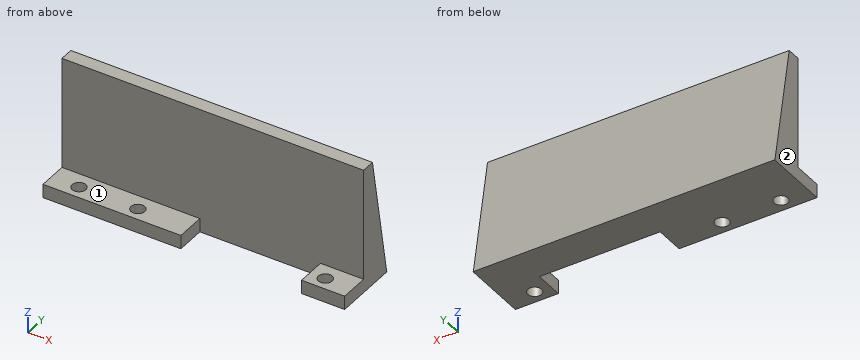
from build123d import *

# Parameters (mm, degrees)
SKETCH1_W           = 70
SKETCH1_H           = 26
BOSS_EXTRUDE1_DEPTH = 3.175
SKETCH2_W           = 70
SKETCH2_H           = 10
BOSS_EXTRUDE2_DEPTH = 3.175
SKETCH3_R           = 1.6
CUT_EXTRUDE1_DEPTH  = 3.175
BOSS_EXTRUDE3_DEPTH = 70
SKETCH5_W           = 28
SKETCH5_H           = 6.825
CUT_EXTRUDE2_DEPTH  = 10


with BuildPart() as part:
    # Sketch1 → Boss-Extrude1 (new body)
    with BuildSketch(Plane(origin=(0, 0, 0), x_dir=(1, 0, 0), z_dir=(0, 1, 0))):
        Rectangle(SKETCH1_W, SKETCH1_H)
    extrude(amount=BOSS_EXTRUDE1_DEPTH)

    # Sketch2 → Boss-Extrude2 (add)
    with BuildSketch(Plane(origin=(0, 0, -13), x_dir=(-1, 0, 0), z_dir=(0, 0, -1))):
        with Locations((0, -1.825)):
            Rectangle(SKETCH2_W, SKETCH2_H)
    extrude(amount=BOSS_EXTRUDE2_DEPTH)

    # Sketch3 → Cut-Extrude1 (cut)
    with BuildSketch(Plane.XY.offset(-13)):
        with Locations((-14.914, -3.825)):
            Circle(SKETCH3_R)
        with Locations((28.575, -3.825)):
            Circle(SKETCH3_R)
        with Locations((-28.575, -3.825)):
            Circle(SKETCH3_R)
    extrude(amount=-CUT_EXTRUDE1_DEPTH, mode=Mode.SUBTRACT)

    # Sketch4 → Boss-Extrude3 (add)
    with BuildSketch(Plane(origin=(35, 0, 0), x_dir=(0, 0, -1), z_dir=(1, 0, 0))):
        Polygon((16.175, 3.175), (16.175, 8.412812241), (16.143192443, 8.313731132), (-13, 3.175), align=None)
    extrude(amount=-BOSS_EXTRUDE3_DEPTH)

    # Sketch5 → Cut-Extrude2 (cut)
    with BuildSketch(Plane(origin=(0, 0, -16.175), x_dir=(-1, 0, 0), z_dir=(0, 0, -1))):
        with Locations((-11, -3.4125)):
            Rectangle(SKETCH5_W, SKETCH5_H)
    extrude(amount=-CUT_EXTRUDE2_DEPTH, mode=Mode.SUBTRACT)


solid = part.part
Could you check a few things on this model? Use its own coordinates, in mm. Face numbers are marked on the shaded views. A direction names the side the tool comes from. Round coordinates to 2 decimals unless told otherwise and drop trailing zeros. Write each loop counter-clockwise with the first axis right and the second up, starting at its lowest first coordinate (ties: lowest second). Pieces come first, ordered by that corner, then holes. Notation, with made-up numbers: (79.5, 49) -> (85.5, 49) arc R22 ccw to (85.5, 58) -> close; hole circle Ø4 at (-29, -10.5). An arc over 180 degrees is marked (long way). Use a Markdown table: item, result.
1. If we section it at C-C (z = 1.75): List the corners of the cut face in (x, y) for me, then the cut area to 3 significant figures.
Answer key:
| item | result |
|---|---|
| outline | (-35, 0) -> (35, 0) -> (35, 5.16) -> (-35, 5.16) -> close |
| area | 361 mm^2 |
2. Which directions (+Z, -Z, +X, -X, +Y, -Y) give clear straight access to the entire face, cutting with the end or side of a thin tool? Please do the marked faces 1 and 2.
Answer key:
| item | result |
|---|---|
| face 1 | +Z, +X, -X, -Y |
| face 2 | +Z, -Z, -X, +Y, -Y |
3. If we section it at D-D (y = 5.75): List the corners of the cut face in (x, z) for me (3 decimals), then the cut area to 3 significant figures.
Answer key:
| item | result |
|---|---|
| outline | (-35, -16.175) -> (35, -16.175) -> (35, -1.604) -> (-35, -1.604) -> close |
| area | 1,020 mm^2 |
4. For pin 1 Ø5 at (x, z) = (-3, -10) entering from +Y; pin 2 Ø5 at (x, y) = (-28.575, -3.825) entering from +Z; pin 3 Ø5 at (x, z) = (10, -6.5) entering from -Y, each with a flat end and sliding along its axis, tell me the tip position at first contact or that it passes through.
Answer key:
| item | result |
|---|---|
| pin 1 | stops at y = 7.67 |
| pin 2 | stops at z = -13 |
| pin 3 | stops at y = 0 |
5. Please list where these lines run through material, in increasing order: probe 1 along Z at (x, y) = (-25.5, -0.25) (3 decimals); probe 2 along Y at (x, z) = (15, -7.5); probe 3 along Y at (x, z) = (31, -6.25).
Answer key:
| item | result |
|---|---|
| probe 1 | z = -16.175 to -13 |
| probe 2 | y = 0 to 6.79 |
| probe 3 | y = 0 to 6.57 |
6. If we section it at B-B (y = -4.5): List the corners of the cut face in (x, z) for me (3 decimals), then the cut area to 3 significant figures.
Answer key:
| item | result |
|---|---|
| outline | (-35, -16.175) -> (-30.026, -16.175) -> (-30.026, -13) -> (-35, -13) -> close; (-27.124, -16.175) -> (-16.365, -16.175) -> (-16.365, -13) -> (-27.124, -13) -> close; (-13.463, -16.175) -> (-3, -16.175) -> (-3, -13) -> (-13.463, -13) -> close; (25, -16.175) -> (27.124, -16.175) -> (27.124, -13) -> (25, -13) -> close; (30.026, -16.175) -> (35, -16.175) -> (35, -13) -> (30.026, -13) -> close |
| area | 106 mm^2 |
7. If we section it at A-A (x = 9): List the corners of the cut face in (y, z) for me (3 decimals), then the cut area to 3 significant figures.
Answer key:
| item | result |
|---|---|
| outline | (0, -16.175) -> (8.413, -16.175) -> (8.314, -16.143) -> (3.175, 13) -> (0, 13) -> close |
| area | 168 mm^2 |
